Check sheet for the modelled part. Datum: model origin and axes. Units: mm. Round coordinates to 2 decimals unless told otherwise and drop trailing zeros. Order: outer loops, then holes, each group sorted by start corner. A loop starts at its lowest first (then second) coordinate and runs counter-clockwise, first axis right, second up.
Q1. Mould release check, pull along Y, two halves, no side actions. Record for faces 1 (the flat face through (-7.715, 2, -14)), 2 (the conical face through (-21.236, 0.138, -24.657)), 3 (the cylindrical face through (-21.501, 2.665, -24.916)): +Y half, -Y half, draft (parallel to the pull), parting line (faces both ways), or undercut.
Q2. Depth check by flat-ended pin: P1, Ø1, axis at y = 2.5, z = -13.5, coming from the +X side. Enter the tip coordinate at first touch or a pass-through.
Q3. Cross-section at B-B on y = 1.7. Record the cut outline in (x, z) (3 decimals).
Q4. Cross-section at A-A on x = 12. Record the cut outline in (y, z) (1 decimal).
Q5. Scan lines: probe 1 along Z at (x, y) = (11.5, 2.35); probe 2 along Y at (x, z) = (-3, -14); probe 3 along Z at (x, y) = (1.5, 3.5). Record each from-to range of solid material in increasing order.
from build123d import *

# Parameters (mm, degrees)
SKETCH1_W           = 44.45
SKETCH1_H           = 51.3588
BOSS_EXTRUDE1_DEPTH = 4.7625
CUT_EXTRUDE1_DEPTH  = 29.94025
FILLET1_R           = 2.54
CHAMFER1_SIZE       = 0.508


with BuildPart() as part:
    # Sketch1 → Boss-Extrude1 (new body)
    with BuildSketch(Plane(origin=(0, 0, 0), x_dir=(1, 0, 0), z_dir=(0, 1, 0))):
        Rectangle(SKETCH1_W, SKETCH1_H)
    extrude(amount=BOSS_EXTRUDE1_DEPTH)

    # Sketch2 → Cut-Extrude1 (cut)
    with BuildSketch(Plane(origin=(22.225, 0, 0), x_dir=(0, 0, -1), z_dir=(1, 0, 0))):
        with BuildLine():
            ThreePointArc((15.757525, 2.38125), (15.292557015, 3.503782015), (14.170025, 3.96875))
            Line((14.170025, 3.96875), (14.170025, 0.79375))
            ThreePointArc((14.170025, 0.79375), (15.292557015, 1.258717985), (15.757525, 2.38125))
        make_face()
        with BuildLine():
            Line((14.170025, 0.79375), (14.170025, 3.96875))
            ThreePointArc((14.170025, 3.96875), (12.582525, 2.38125), (14.170025, 0.79375))
        make_face()
    extrude(amount=-CUT_EXTRUDE1_DEPTH, mode=Mode.SUBTRACT)

    # Fillet1
    fillet1_edges = [part.edges().sort_by_distance(p)[0] for p in [
        (-22.225, 2.38125, -25.6794),
        (-22.225, 2.38125, 25.6794),
    ]]
    fillet(fillet1_edges, radius=FILLET1_R)

    # Chamfer1
    chamfer1_edges = [part.edges().sort_by_distance(p)[0] for p in [
        (-22.225, 0, 0),
        (1.27, 0, 25.6794),
        (-21.481051224, 0, 24.935451224),
        (-21.481051224, 0, -24.935451224),
        (1.27, 0, -25.6794),
        (22.225, 0, 0),
    ]]
    chamfer(chamfer1_edges, length=CHAMFER1_SIZE)


solid = part.part
Results found:
1. face 1: undercut
1. face 2: -Y half
1. face 3: draft
2. P1: stops at x = -7.72
3. outline: (-22.225, -23.139) arc R2.54 ccw to (-19.685, -25.679) - (22.225, -25.679) - (22.225, -15.604) - (-7.715, -15.604) - (-7.715, -12.736) - (22.225, -12.736) - (22.225, 25.679) - (-19.685, 25.679) arc R2.54 ccw to (-22.225, 23.139) - close
4. outline: (0, -25.2) - (0.5, -25.7) - (4.8, -25.7) - (4.8, 25.7) - (0.5, 25.7) - (0, 25.2) - close; hole circle Ø3.2 at (2.4, -14.2)
5. probe 1: z = -25.68 to -15.76, -12.58 to 25.68
5. probe 2: y = 0 to 0.8, 3.96 to 4.76
5. probe 3: z = -25.68 to -15.3, -13.04 to 25.68
